from build123d import *

# Parameters (mm, degrees)
BOSS_EXTRUDE1_DEPTH = 10
SHELL1_T            = -1.25
FILLET1_R           = 2.5
CHAMFER1_SIZE       = 1.25


with BuildPart() as part:
    # Sketch1 → Boss-Extrude1 (new body)
    with BuildSketch(Plane(origin=(0, 0, 0), x_dir=(1, 0, 0), z_dir=(0, 1, 0))):
        with BuildLine():
            Line((-47.5, -30), (47.5, -30))
            ThreePointArc((47.5, -30), (49.267766953, -29.267766953), (50, -27.5))
            Line((50, -27.5), (50, 27.5))
            ThreePointArc((50, 27.5), (49.267766953, 29.267766953), (47.5, 30))
            Line((47.5, 30), (-47.5, 30))
            ThreePointArc((-47.5, 30), (-49.267766953, 29.267766953), (-50, 27.5))
            Line((-50, 27.5), (-50, -27.5))
            ThreePointArc((-50, -27.5), (-49.267766953, -29.267766953), (-47.5, -30))
        make_face()
    extrude(amount=BOSS_EXTRUDE1_DEPTH)

    # Shell1
    shell1_openings = [part.faces().sort_by_distance(p)[0] for p in [
        (0, 0, 0),
    ]]
    offset(amount=SHELL1_T, openings=shell1_openings, kind=Kind.INTERSECTION)

    # Fillet1
    fillet1_edges = [part.edges().sort_by_distance(p)[0] for p in [
        (49.267766953, 10, 29.267766953),
        (50, 10, 0),
        (49.267766953, 10, -29.267766953),
        (0, 10, -30),
        (-49.267766953, 10, -29.267766953),
        (-50, 10, 0),
        (-49.267766953, 10, 29.267766953),
        (0, 10, 30),
    ]]
    fillet(fillet1_edges, radius=FILLET1_R)

    # Chamfer1
    chamfer1_edges = [part.edges().sort_by_distance(p)[0] for p in [
        (-48.383883476, 0, 28.383883476),
        (0, 0, 28.75),
        (48.383883476, 0, 28.383883476),
        (48.75, 0, 0),
        (48.383883476, 0, -28.383883476),
        (0, 0, -28.75),
        (-48.383883476, 0, -28.383883476),
        (-48.75, 0, 0),
    ]]
    chamfer(chamfer1_edges, length=CHAMFER1_SIZE - 0.0001)  # a hair under: the kernel refuses the full size


solid = part.part
Work out the finished part from the listing and answer in its coordinate system (mm). A direction names the side the tool comes from. Round coordinates to 2 decimals unless told otherwise and drop trailing zeros. Write each loop counter-clockwise with the first axis right and the second up, starting at its lowest first coordinate (ties: lowest second). Pieces come first, ordered by that corner, then holes. Notation, with made-up numbers: (10.5, 49) - (56.5, 49) arc R27 ccw to (56.5, 75) - close; hole circle Ø1 at (69.5, -14.5). An arc over 180 degrees is marked (long way). Answer in a Markdown table with one row per item. Add a question column.
1. The mould has two halves that part along X. Classify faces 1 (the flat face through (-1, 5, 28.75)), 2 (the cylindrical face through (-0.665, 9.248, -29.287)), 3 (the flat face through (-50, 4, 0)): +X half, -X half, draft (parallel to the pull), parting line (faces both ways), or undercut.
2. Find the intervals of material crossed by line 1 along X through (y, z) = (2, 5); line 2 along Z through (x, y) = (13.5, 6), in increasing order. Write a range as from..to.
3. Given pin 1 (8 mm diameter, centred on x = -36.5, z = 12, fed in from -Y), flat-ended and moving along its own axis, determine where the tip first touches the part or whether it passes through.
4. A cutting plane is placed at A-A, the plane y = 4. Determine the outline of the cut face in (x, z), and give its area (3 significant figures).
5. For faces 4 (the flat face through (48.75, 5, 0)), 5 (the cylindrical face through (49.248, 3.698, 29.287)), determine the directions among +Z, -Z, +X, -X, +Y, -Y from which every point of the face is accessible in a straight line to the end or side of a thin tool.
Worked out:
| question | item | result |
|---|---|---|
| 1 | face 1 | undercut |
| 1 | face 2 | draft |
| 1 | face 3 | -X half |
| 2 | line 1 | -50..-48.75, 48.75..50 |
| 2 | line 2 | -30..-28.75, 28.75..30 |
| 3 | pin 1 | y = 8.75 |
| 4 | outline | (-50, -27.5) arc R2.5 ccw to (-47.5, -30) - (47.5, -30) arc R2.5 ccw to (50, -27.5) - (50, 27.5) arc R2.5 ccw to (47.5, 30) - (-47.5, 30) arc R2.5 ccw to (-50, 27.5) - close; hole (-48.75, -27.5) arc R1.25 ccw to (-47.5, -28.75) - (47.5, -28.75) arc R1.25 ccw to (48.75, -27.5) - (48.75, 27.5) arc R1.25 ccw to (47.5, 28.75) - (-47.5, 28.75) arc R1.25 ccw to (-48.75, 27.5) - close |
| 4 | area | 390 mm^2 |
| 5 | face 4 | -Y |
| 5 | face 5 | +Z, +X, +Y, -Y |
